Source: CAD feature listing. Evaluate the final solid. Frame: model axes, mm. A direction names the side the tool comes from. Round coordinates to 2 decimals unless told otherwise and drop trailing zeros. Loops run counter-clockwise (first coordinate to the right, second up) from the corner with the lowest first, then second, coordinate; pieces in that order, holes last. Notation, with made-up numbers: M 10.5,21 L 25.5,21 A9 ccw 25.5,28 Z; hole C 44.25,28 d9. An arc over 180 degrees is marked long. Write each question's results on one line, items separated by ' | '. Start each with the question number.
1. Contact query for flat-ended pins moving along their axis: pin 1 Ø4.5 at (x, z) = (0, 12) entering from -Y; pin 2 Ø3.5 at (x, z) = (0, 24) entering from +Y; pin 3 Ø4 at (y, z) = (-9, 6) entering from +X. Output: stop coordinate, or through.
2. Section D-D on z = 24. Output: boundary loops of the cut face in (x, y), and give its area (3 significant figures).
3. Section B-B on x = 0. Output: boundary loops of the cut face in (y, z).
4. Section C-C on y = -4. Output: boundary loops of the cut face in (x, z), and give its area (3 significant figures).
5. Ray query, line 1 (Z direction, x = 0, y = -2.25); line 2 (Z direction, x = 0, y = -17.75); line 3 (Z direction, x = -1.5, y = -9). Return the intervals inside material, ascending.
6. Section A-A on y = -9. Output: boundary loops of the cut face in (x, z), and give its area (3 significant figures).
7. Draft query along X for faces 3 (the cylindrical face through (-0.46, -17.49, 20.53)), 4 (the flat face through (8.5, -8.4, 0.5)), 5 (the flat face through (-1, -8, 30)). Return one class per face: released by +X, released by -X, zero draft, split by the parting line, or undercut.
8. Set-up query: faces 1 (the cylindrical face through (-1.432, -8.759, 19.834)), 2 (the cylindrical face through (-0.759, -17.493, 15.417)). Return all of +Z, -Z, +X, -X, +Y, -Y with unobstructed straight access to the full face (end or side cutting, diameter ignored); none if empty.
from build123d import *

# Parameters (mm, degrees)
F0_W           = 18
F0_H           = 30
F1_DEPTH       = 18
F4_D           = 7
F4_DEPTH       = 1.001
F5_D           = 3.7
F5_CSINK_D     = 7
F5_CSINK_ANGLE = 90
F8_D           = 7
F8_DEPTH       = 1.001
F9_D           = 3.7
F9_CSINK_D     = 7
F9_CSINK_ANGLE = 90
F10_SIZE       = 1


with BuildPart() as f1:
    # F0 (on Front) → F1 (new body)
    with BuildSketch(Plane.XZ):
        with Locations((0, 15)):
            Rectangle(F0_W, F0_H)
    extrude(amount=F1_DEPTH)

    # F4 (through all, one way)
    with BuildSketch(Plane(origin=(0, -17, 0), x_dir=(1, 0, 0), z_dir=(0, 1, 0))):
        with Locations((0, -24), (0, -12)):
            Circle(F4_D / 2)
    extrude(amount=-F4_DEPTH, mode=Mode.SUBTRACT)

    # F5 (through all)
    with Locations(Plane.XZ.offset(17)):
        with Locations((0, 24), (0, 12)):
            CounterSinkHole(F5_D / 2, F5_CSINK_D / 2, counter_sink_angle=F5_CSINK_ANGLE)

    # F8 (through all, one way)
    with BuildSketch(Plane(origin=(8, 0, 0), x_dir=(0, 1, 0), z_dir=(-1, 0, 0))):
        with Locations((-9, -18), (-9, -6)):
            Circle(F8_D / 2)
    extrude(amount=-F8_DEPTH, mode=Mode.SUBTRACT)

    # F9 (through all)
    with Locations(Plane.YZ.offset(8)):
        with Locations((-9, 18), (-9, 6)):
            CounterSinkHole(F9_D / 2, F9_CSINK_D / 2, counter_sink_angle=F9_CSINK_ANGLE)

    # F10
    f10_edges = [f1.edges().sort_by_distance(p)[0] for p in [
        (9, -18, 15),
        (9, -9, 30),
        (0, -18, 30),
        (9, -9, 0),
        (0, -18, 0),
    ]]
    chamfer(f10_edges, length=F10_SIZE)


solid = f1.part
Taken from the geometry:
1) pin 1: y = -15.75 | pin 2: through | pin 3: x = 6.5
2) outline: M -9,-18 L -3.5,-18 L -3.5,-17 L -1.85,-15.35 L -1.85,0 L -9,0 Z; M 1.85,-15.35 L 3.5,-17 L 3.5,-18 L 8,-18 L 9,-17 L 9,0 L 1.85,0 Z | area: 251 mm^2
3) outline: M -18,1 L -17,0 L 0,0 L 0,10.15 L -15.35,10.15 L -17,8.5 L -18,8.5 Z; M -18,15.5 L -17,15.5 L -15.35,13.85 L 0,13.85 L 0,22.15 L -15.35,22.15 L -17,20.5 L -18,20.5 Z; M -18,27.5 L -17,27.5 L -15.35,25.85 L 0,25.85 L 0,30 L -17,30 L -18,29 Z; hole C -9,6 d3.7; hole C -9,18 d3.7
4) outline: M -9,0 L 8,0 L 9,1 L 9,29 L 8,30 L -9,30 Z; hole C 0,12 d3.7; hole C 0,24 d3.7 | area: 517 mm^2
5) line 1: 0 to 10.15, 13.85 to 22.15, 25.85 to 30 | line 2: 0.75 to 8.5, 15.5 to 20.5, 27.5 to 29.25 | line 3: 0 to 4.15, 7.85 to 10.92, 13.08 to 16.15, 19.85 to 22.92, 25.08 to 30
6) outline: M -9,0 L 8,0 L 9,1 L 9,2.5 L 8,2.5 L 6.35,4.15 L -9,4.15 Z; M -9,7.85 L 6.35,7.85 L 8,9.5 L 9,9.5 L 9,14.5 L 8,14.5 L 6.35,16.15 L -9,16.15 Z; M -9,19.85 L 6.35,19.85 L 8,21.5 L 9,21.5 L 9,29 L 8,30 L -9,30 Z; hole C 0,12 d3.7; hole C 0,24 d3.7 | area: 372 mm^2
7) face 3: undercut | face 4: released by +X | face 5: zero draft
8) face 1: +X, -X | face 2: -Y
